Geometry check sheet. Reference: drawing and pictorial views, mm from the part's lowest x, y, z. Round coordinates to 2 decimals unless told otherwise and drop trailing zeros. Order: outer loops, then holes, each group sorted by start corner. A loop starts at its lowest first (then second) coordinate and runs counter-clockwise, first axis right, second up.
Q1. Scan lines: probe 1 along X at (y, z) = (147.5, 7.5); probe 2 along Y at (x, z) = (160.5, 10.5). Record each from-to range of solid material in increasing order.
Q2. Cross-section at B-B on z = 8.5. Record the cut outline in (x, y), then the cut area to 3 significant figures.
Q3. Cross-section at A-A on y = 60.5. Record the cut outline in (x, z).
Q4. Depth check by flat-ended pin: P1, Ø5, axis at y = 221, z = 9, coming from the -X side; P2, Ø5, axis at x = 184, z = 10, coming from the -Y side; P3, Ø6.5, axis at x = 182, z = 9.5, coming from the +Y side. Enter the tip coordinate at first touch or a pass-through.
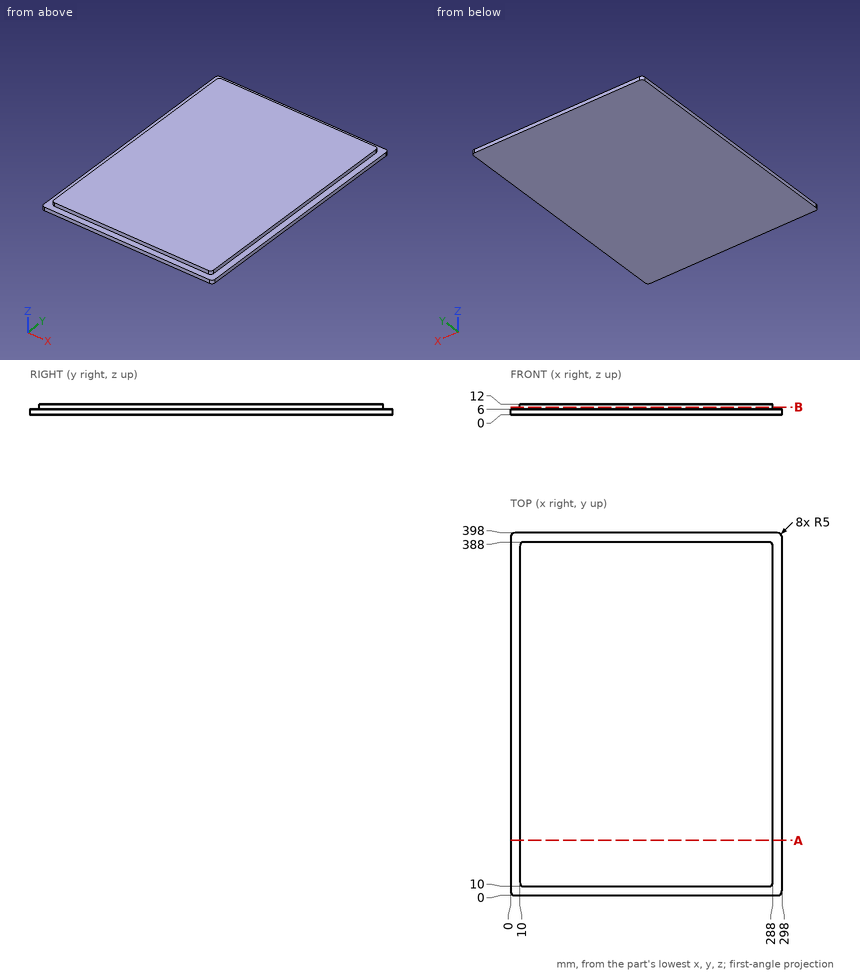
Results found:
1. probe 1: x = 10 to 288
1. probe 2: y = 10 to 388
2. outline: (10, 15) arc R5 ccw to (15, 10) - (283, 10) arc R5 ccw to (288, 15) - (288, 383) arc R5 ccw to (283, 388) - (15, 388) arc R5 ccw to (10, 383) - close
2. area: 105,000 mm2
3. outline: (0, 0) - (298, 0) - (298, 6) - (288, 6) - (288, 12) - (10, 12) - (10, 6) - (0, 6) - close
4. P1: stops at x = 10
4. P2: stops at y = 10
4. P3: stops at y = 388
